from build123d import *


with BuildPart() as part:
    # Sketch2 → Revolve1 (revolve)
    with BuildSketch(Plane.XY, mode=Mode.PRIVATE) as revolve1_sk:
        Polygon((24.875666667, 0), (68.535, 0), (68.535, 52.035833333), (55.335666667, 52.035833333), (63.536435897, 66.2505), (0, 66.2505), (0, 0), align=None)
    revolve(revolve1_sk.sketch.rotate(Axis((0, 0, 0), (0, 1, 0)), 90), axis=Axis((0, 0, 0), (0, 1, 0)))

    # Sketch3 → Revolve2 (revolve)
    with BuildSketch(Plane.XY, mode=Mode.PRIVATE) as revolve2_sk:
        with BuildLine():
            Line((80.92907592, 94.620601836), (72.088666667, 70.8195))
            Line((72.088666667, 70.8195), (73.8655, 70.8195))
            Line((73.8655, 70.8195), (70.928285714, 66.2505))
            Line((70.928285714, 66.2505), (0, 66.2505))
            Line((0, 66.2505), (0, 109.909833333))
            Line((0, 109.909833333), (88.334, 109.909833333))
            ThreePointArc((88.334, 109.909833333), (84.396122366, 102.379234735), (80.92907592, 94.620601836))
        make_face()
    revolve(revolve2_sk.sketch.rotate(Axis((0, 0, 0), (0, 1, 0)), 90), axis=Axis((0, 0, 0), (0, 1, 0)))

    # Sketch5 → Revolve3 (revolve)
    with BuildSketch(Plane.XY, mode=Mode.PRIVATE) as revolve3_sk:
        Polygon((0, 109.909833333), (113.4635, 109.909833333), (113.4635, 119.5555), (135.039333333, 119.5555), (135.039333333, 123.363), (0, 123.363), align=None)
    revolve(revolve3_sk.sketch.rotate(Axis((0, 0, 0), (0, 1, 0)), 90), axis=Axis((0, 0, 0), (0, 1, 0)))


solid = part.part
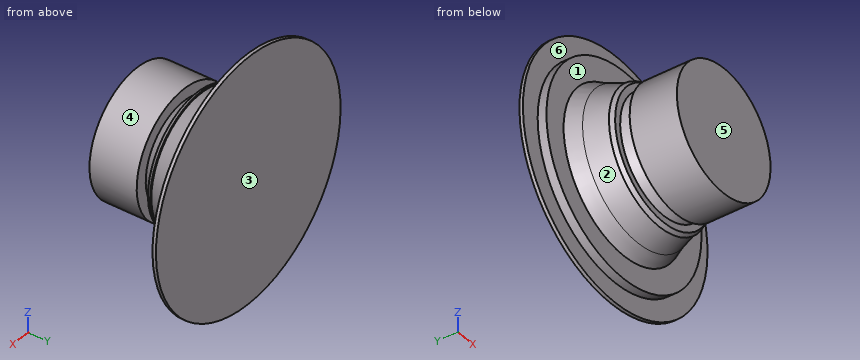
Could you check a few things on this model? Use its own coordinates, in mm. Face numbers are marked on the shaded views. A direction names the side the tool comes from. Give positions to 0.01 mm unless a question says otherwise; leave off trailing zeros. Order: outer loops, then holes, each group sorted by start corner. A loop starts at its lowest first (then second) coordinate and runs counter-clockwise, first axis right, second up.
Item 1: I need wall thicknesses on line 1 (Y direction, x = -14.5, z = -62); line 2 (Y direction, x = -79, z = -66.5); line 3 (Y direction, x = 116, z = 65.5). Which ranges of each line are inside material? Lowest first, please.
Item 2: If we section it at A-A, the plane y = 14: Write out the boundary of the cut face in (x, z) (3 decimals), plus the area to 3 significant figures.
Item 3: If we section it at B-B, the plane x = -105: Write out the boundary of the cut face in (y, z).
Item 4: If we section it at D-D, the plane x = 0: Write out the boundary of the cut face in (y, z) (1 decimal).
Item 5: If we section it at C-C, the plane z = 0: Write out the boundary of the cut face in (x, y) (1 decimal).
Item 6: For the marked faces 5 and 6, which set-ups out of +Z, -Z, +X, -X, +Y, -Y let a thin tool reach every point of the face, with its end or its side?
Item 7: I'm going to push flat-ended pins straight in: pin 1 (5 mm diameter, centred on x = -26.5, y = 84.5, fed in from -Z); pin 2 (12 mm diameter, centred on x = -7.5, y = 15.5, fed in from -Z); pin 3 (5 mm diameter, centred on x = -28.5, y = 58, fed in from -Z). Where does each tip first touch, or does it pass through?
Item 8: If we mould it in two halves opening along Y, with no side actions, what happens to the marked faces 1, 2, 3 and 4? For each: pulls with the +Y half, pulls with the -Y half, needs draft (parallel to the pull), parting line crosses it, or undercut.
Values:
1. line 1: y = 0 to 52.04, 66.25 to 123.36
1. line 2: y = 109.91 to 123.36
1. line 3: y = 119.56 to 123.36
2. outline: circle Ø137.07 at (0, 0)
2. area: 14,800 mm2
3. outline: (109.91, -43) - (119.56, -43) - (119.56, -84.92) - (123.36, -84.92) - (123.36, 84.92) - (119.56, 84.92) - (119.56, 43) - (109.91, 43) - close
4. outline: (0, -68.5) - (52, -68.5) - (52, -55.3) - (66.3, -63.5) - (66.3, -70.9) - (70.8, -73.9) - (70.8, -72.1) - (94.6, -80.9) arc R138 cw to (109.9, -88.3) - (109.9, -113.5) - (119.6, -113.5) - (119.6, -135) - (123.4, -135) - (123.4, 135) - (119.6, 135) - (119.6, 113.5) - (109.9, 113.5) - (109.9, 88.3) arc R138 cw to (94.6, 80.9) - (70.8, 72.1) - (70.8, 73.9) - (66.3, 70.9) - (66.3, 63.5) - (52, 55.3) - (52, 68.5) - (0, 68.5) - close
5. outline: (-135, 119.6) - (-113.5, 119.6) - (-113.5, 109.9) - (-88.3, 109.9) arc R138 cw to (-80.9, 94.6) - (-72.1, 70.8) - (-73.9, 70.8) - (-70.9, 66.3) - (-63.5, 66.3) - (-55.3, 52) - (-68.5, 52) - (-68.5, 0) - (68.5, 0) - (68.5, 52) - (55.3, 52) - (63.5, 66.3) - (70.9, 66.3) - (73.9, 70.8) - (72.1, 70.8) - (80.9, 94.6) arc R138 cw to (88.3, 109.9) - (113.5, 109.9) - (113.5, 119.6) - (135, 119.6) - (135, 123.4) - (-135, 123.4) - close
6. face 5: +Z, -Z, +X, -X, -Y
6. face 6: -Y
7. pin 1: stops at z = -73.8
7. pin 2: stops at z = -68.52
7. pin 3: stops at z = -53.5
8. face 1: pulls with the -Y half
8. face 2: undercut
8. face 3: pulls with the +Y half
8. face 4: needs draft
